from build123d import *

# Parameters (mm, degrees)
EXTRUDE_1_DEPTH      = 16
EXTRUDE_1_DEPTH_BACK = 16
SKETCH_1_R           = 37.5
SKETCH_1_R_2         = 24
EXTRUDE_2_DEPTH      = 18
EXTRUDE_2_DEPTH_BACK = 18
SKETCH_1_3_R         = 24
EXTRUDE_3_DEPTH      = 24
EXTRUDE_3_DEPTH_BACK = 24
SKETCH_2_R           = 15
EXTRUDE_4_DEPTH      = 3
EXTRUDE_5_REACH      = 93.722
SKETCH_3_W           = 60
SKETCH_3_H           = 3
EXTRUDE_6_DEPTH      = 5
SKETCH_5_R           = 21
EXTRUDE_7_DEPTH      = 2
SKETCH_5_3_W         = 93
SKETCH_5_3_H         = 63
SKETCH_5_3_R         = 21
EXTRUDE_8_DEPTH      = 2
FILLET_1_R           = 10
FILLET_2_R           = 10
FILLET_3_R           = 10


with BuildPart() as part:
    # Sketch 1 → Extrude 1 (new, two sides: drawn at the far end of the back side and taken through both)
    with BuildSketch(Plane.XY.offset(-EXTRUDE_1_DEPTH_BACK)):
        Circle(SKETCH_1_R)
        Circle(SKETCH_1_R_2, mode=Mode.SUBTRACT)
    extrude(amount=EXTRUDE_1_DEPTH + EXTRUDE_1_DEPTH_BACK)

    # Sketch 1_3 → Extrude 2 (add, two sides: drawn at the far end of the back side and taken through both)
    with BuildSketch(Plane.XY.offset(-EXTRUDE_2_DEPTH_BACK)):
        Circle(SKETCH_1_3_R)
        Polygon((6.927335766, 0.109632038), (3.368723753, 6.054064773), (-3.558612013, 5.944432735), (-6.927335766, -0.109632038), (-3.368723753, -6.054064773), (3.558612013, -5.944432735), align=None, mode=Mode.SUBTRACT)
    extrude(amount=EXTRUDE_2_DEPTH + EXTRUDE_2_DEPTH_BACK)

    # Sketch 1_4 → Extrude 3 (add, two sides: drawn at the far end of the back side and taken through both)
    with BuildSketch(Plane.XY.offset(-EXTRUDE_3_DEPTH_BACK)):
        Polygon((3.558612013, -5.944432735), (6.927335766, 0.109632038), (3.368723753, 6.054064773), (-3.558612013, 5.944432735), (-6.927335766, -0.109632038), (-3.368723753, -6.054064773), align=None)
    extrude(amount=EXTRUDE_3_DEPTH + EXTRUDE_3_DEPTH_BACK)

    # Sketch 2 → Extrude 4 (add)
    # profile 1 of 3: a face of its own
    with BuildSketch(Plane.XY.offset(18)):
        with BuildLine():
            Line((-15, 68), (-15, 18.734993995))
            ThreePointArc((-15, 18.734993995), (5.780513413, 23.293468284), (22.018813536, 9.548395178))
            Line((22.018813536, 9.548395178), (42.679560047, 48.612635579))
            ThreePointArc((42.679560047, 48.612635579), (44.41122357, 53.146110919), (45, 57.96320543))
            Line((45, 57.96320543), (45, 68))
            Line((45, 68), (0, 68))
            Line((0, 68), (-15, 68))
        make_face()
    # profile 2 of 3: a face of its own
    with BuildSketch(Plane.XY.offset(18)):
        with BuildLine():
            Line((-15, 18.734993995), (-15, 0))
            ThreePointArc((-15, 0), (0, 15), (15, 0))
            ThreePointArc((15, 0), (14.558417677, -3.612820883), (13.259670035, -7.012927388))
            Line((13.259670035, -7.012927388), (22.018813536, 9.548395178))
            ThreePointArc((22.018813536, 9.548395178), (5.780513413, 23.293468284), (-15, 18.734993995))
        make_face()
    # profile 3 of 3: a face of its own
    with BuildSketch(Plane.XY.offset(18)):
        Circle(SKETCH_2_R)
        Polygon((-3.558612013, 5.944432735), (3.368723753, 6.054064773), (6.927335766, 0.109632038), (3.558612013, -5.944432735), (-3.368723753, -6.054064773), (-6.927335766, -0.109632038), align=None, mode=Mode.SUBTRACT)
    extrude_4 = extrude(amount=EXTRUDE_4_DEPTH)

    # Mirror 1: Extrude 4 across plane
    add(extrude_4.mirror(Plane.XY))

    # Sketch 3 → Extrude 5 (add, up to next)
    with BuildSketch(Plane(origin=(0, 0, 18), x_dir=(-1, 0, 0), z_dir=(0, 0, -1)), mode=Mode.PRIVATE) as extrude_5_sk1:
        with Locations((-15, 66.5)):
            Rectangle(SKETCH_3_W, SKETCH_3_H)
    extrude_5_tool1 = extrude(extrude_5_sk1.sketch, amount=EXTRUDE_5_REACH, mode=Mode.PRIVATE) - part.part
    add(extrude_5_tool1.solids().sort_by_distance((15, 66.5, 18))[0])

    # Sketch 4 → Extrude 6 (add)
    with BuildSketch(Plane(origin=(0, 68, 0), x_dir=(1, 0, 0), z_dir=(0, 1, 0))):
        with BuildLine():
            ThreePointArc((24, 21), (9.150757595, 14.849242405), (3, 0))
            Line((3, 0), (45, 0))
            ThreePointArc((45, 0), (38.849242405, 14.849242405), (24, 21))
        make_face()
        with BuildLine():
            Line((45, 0), (3, 0))
            ThreePointArc((3, 0), (9.150757581, -14.849242391), (23.999999961, -21))
            ThreePointArc((23.999999961, -21), (38.849242391, -14.849242419), (45, 0))
        make_face()
    extrude(amount=EXTRUDE_6_DEPTH)

    # Sketch 5 → Extrude 7 (add)
    with BuildSketch(Plane(origin=(0, 73, 0), x_dir=(1, 0, 0), z_dir=(0, 1, 0))):
        with Locations(Location((24, 0, 0), (0, 0, 270))):
            Circle(SKETCH_5_R)
    extrude(amount=EXTRUDE_7_DEPTH)

    # Sketch 5_3 → Extrude 8 (add)
    with BuildSketch(Plane(origin=(0, 73, 0), x_dir=(1, 0, 0), z_dir=(0, 1, 0))):
        with Locations((24, 0)):
            Rectangle(SKETCH_5_3_W, SKETCH_5_3_H)
        with Locations(Location((24, 0, 0), (0, 0, 270))):
            Circle(SKETCH_5_3_R, mode=Mode.SUBTRACT)
    extrude(amount=EXTRUDE_8_DEPTH)

    # Fillet 1
    fillet_1_edges = [part.edges().sort_by_distance(p)[0] for p in [
        (70.5, 74, 31.5),
        (70.5, 74, -31.5),
        (-22.5, 74, -31.5),
        (-22.5, 74, 31.5),
    ]]
    fillet(fillet_1_edges, radius=FILLET_1_R)

    # Fillet 2
    fillet_2_edges = [part.edges().sort_by_distance(p)[0] for p in [
        (-37.5, 0, 16),
    ]]
    fillet(fillet_2_edges, radius=FILLET_2_R)

    # Fillet 3
    fillet_3_edges = [part.edges().sort_by_distance(p)[0] for p in [
        (-37.5, 0, -16),
    ]]
    fillet(fillet_3_edges, radius=FILLET_3_R)


solid = part.part
The model under review builds one solid part; all positions refer to its coordinate system, in mm. A direction names the side the tool comes from. Give positions to 0.01 mm unless a question says otherwise; leave off trailing zeros. Order: outer loops, then holes, each group sorted by start corner. A loop starts at its lowest first (then second) coordinate and runs counter-clockwise, first axis right, second up. Notation, with made-up numbers: (15.25, -3.5) -> (28.25, -3.5) arc R18 ccw to (28.25, 21.5) -> close; hole circle Ø5 at (67.5, 65). An arc over 180 degrees is marked (long way). Write item = value, one per line. Start each with the question number.
(1) For pin 1 Ø13 at (x, y) = (0, -13) entering from +Z; pin 2 Ø2 at (y, z) = (-5, 5) entering from +X; pin 3 Ø18 at (x, y) = (1, 41) entering from -Z, all flat-tipped, find the tip position at first contact; note any pin that passes through.
(2) Take a section at B-B (x = 40.5). Write out the cut boundary in (y, z), plus the area to 3 significant figures.
(3) Take a section at A-A (z = -8). Write out the cut boundary in (x, y), plus the area to 3 significant figures.
(4) Take a section at C-C (x = 0). State how many separate pieces and enclosed holes the cut face has, plus the area to 3 significant figures.
(5) For L1, parallel to Z at x = 11.5, y = 29; L2, parallel to Y at x = -14.5, z = -4; L3, parallel to Y at x = 64, z = 12, list the stretches that pass through material, from the lowest coordinate up. Write a range as from..to.
(6) Draft analysis for pull direction Y (two halves, no side actions). For faces 5 (the flat face through (15, 44, -18)), 6 (the flat face through (-11, -12, -18)), 7 (the cylindrical face through (-3.88, -14.49, -19.48)), state which applies: +Y half, -Y half, draft (parallel to the pull), parting line (faces both ways), or undercut.
(7) Tool access review of faces 1 (the flat face through (-5.22, 2.96, -22.52)), 2 (the flat face through (5.22, -2.96, 22.48)), 3 (the flat face through (41, 68, 16)), 4 (the cylindrical face through (-23.977, 1.055, -17.014)): name each direction out of +Z, -Z, +X, -X, +Y, -Y from which nothing blocks a thin tool from reaching the whole face with its end or side.
(8) Take a section at D-D (z = 10). Write out the cut boundary in (x, y).
Returned:
q1.pin_1 = 21
q1.pin_2 = 37.29
q1.pin_3 = -21
q2.outline = (44.49, -21) -> (68, -21) -> (68, -12.99) -> (73, -12.99) -> (73, -31.5) -> (75, -31.5) -> (75, 31.5) -> (73, 31.5) -> (73, 12.99) -> (68, 12.99) -> (68, 21) -> (44.49, 21) -> (44.49, 18) -> (65, 18) -> (65, -18) -> (44.49, -18) -> close
q2.area = 505 mm²
q3.outline = circle Ø74.6 at (0, 0); (-22.5, 73) -> (4.58, 73) -> (4.58, 68) -> (-15, 68) -> (-15, 65) -> (45, 65) -> (45, 68) -> (43.42, 68) -> (43.42, 73) -> (70.5, 73) -> (70.5, 75) -> (-22.5, 75) -> close
q3.area = 4,930 mm²
q4.separate_pieces = 2
q4.enclosed_holes = 1
q4.area = 3,310 mm²
q5.L1 = -21..-18, -15.29..15.29, 18..21
q5.L2 = -34.58..34.58, 65..68, 73..75
q5.L3 = 73..75
q6.face_5 = undercut
q6.face_6 = draft
q6.face_7 = -Y half
q7.face_1 = -Z, -X
q7.face_2 = +Z, +X, -Y
q7.face_3 = +Z, +X
q7.face_4 = none
q8.outline = circle Ø73.33 at (0, 0); (-22.5, 73) -> (5.53, 73) -> (5.53, 68) -> (-15, 68) -> (-15, 65) -> (45, 65) -> (45, 68) -> (42.47, 68) -> (42.47, 73) -> (70.5, 73) -> (70.5, 75) -> (-22.5, 75) -> close
